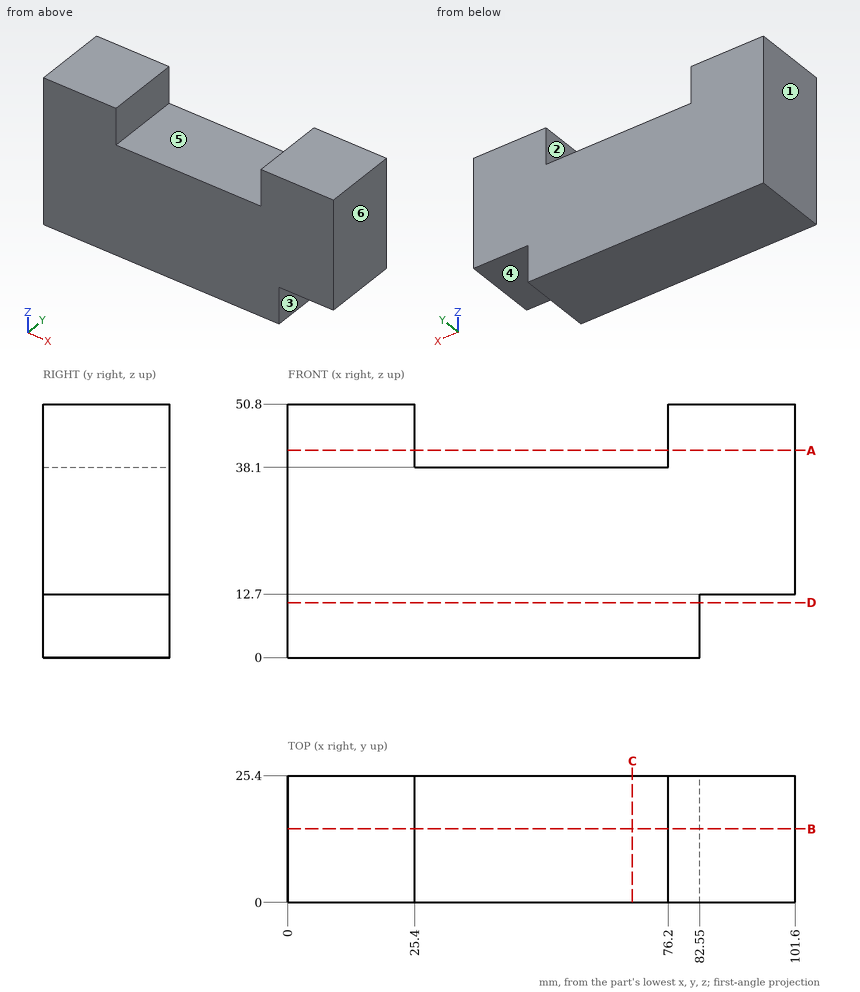
Input: dimensioned drawing with shaded views. Units: mm. Origin: part minimum x, y, z. A direction names the side the tool comes from. Round coordinates to 2 decimals unless told otherwise and drop trailing zeros. Order: outer loops, then holes, each group sorted by start corner. A loop starts at its lowest first (then second) coordinate and runs counter-clockwise, first axis right, second up. Notation, with made-up numbers: (-3.75, 36.25) -> (33.25, 36.25) arc R26 ccw to (33.25, 70.25) -> close; hole circle Ø5 at (-37.5, 23). An arc over 180 degrees is marked (long way). One line per item, written item: value. Start each with the question number.
Q1. Draft query along X for the marked faces 1, 2 and 3. Return one class per face: pulls with the +X half, pulls with the -X half, needs draft (parallel to the pull), parting line crosses it, or undercut.
Q2. Section query B-B (y = 14.75). Return the cut outline in (x, z), plus the area to 3 significant figures.
Q3. Section query A-A (z = 41.5). Return the cut outline in (x, y).
Q4. Access query for the marked faces 4, 5 and 6. Directions: +Z, -Z, +X, -X, +Y, -Y. A direction counts if a zero-diameter tool reaches every point of the face in a straight line with its end or side. Return the directions, or none.
Q5. Material intervals for probe 1 along X at (y, z) = (14.5, 38.5); probe 2 along Z at (x, y) = (90, 10.25); probe 3 along Z at (x, y) = (43, 2.25), sorted ascending.
Q6. Pin query (flat end, axial travel): pin 1 (1 mm diameter, centred on x = 48, y = 21, fed in from +Z); pin 2 (4 mm diameter, centred on y = 12.5, z = 3.5, fed in from +X); pin 3 (5.5 mm diameter, centred on x = 89.5, y = 14.5, fed in from -Z). Return the tip coordinate at first contact, or that it passes through.
Q7. Section query D-D (z = 11). Return the cut outline in (x, y).
Q8. Section query C-C (x = 69). Return the cut outline in (y, z), plus the area to 3 significant figures.
Findings below:
1. face 1: pulls with the -X half
1. face 2: undercut
1. face 3: pulls with the +X half
2. outline: (0, 0) -> (82.55, 0) -> (82.55, 12.7) -> (101.6, 12.7) -> (101.6, 50.8) -> (76.2, 50.8) -> (76.2, 38.1) -> (25.4, 38.1) -> (25.4, 50.8) -> (0, 50.8) -> close
2. area: 4,270 mm²
3. outline: (0, 0) -> (25.4, 0) -> (25.4, 25.4) -> (0, 25.4) -> close; (76.2, 0) -> (101.6, 0) -> (101.6, 25.4) -> (76.2, 25.4) -> close
4. face 4: -Z, +X, +Y, -Y
4. face 5: +Z, +Y, -Y
4. face 6: +Z, -Z, +X, +Y, -Y
5. probe 1: 0 to 25.4, 76.2 to 101.6
5. probe 2: 12.7 to 50.8
5. probe 3: 0 to 38.1
6. pin 1: z = 38.1
6. pin 2: x = 82.55
6. pin 3: z = 12.7
7. outline: (0, 0) -> (82.55, 0) -> (82.55, 25.4) -> (0, 25.4) -> close
8. outline: (0, 0) -> (25.4, 0) -> (25.4, 38.1) -> (0, 38.1) -> close
8. area: 968 mm²
